Design review of the part shown in the three views and the two pictorial views. Dimensions are in mm from the part's minimum x, y and z. Coordinates: 2 decimals unless noted, no trailing zeros. Loops run counter-clockwise (first coordinate to the right, second up) from the corner with the lowest first, then second, coordinate; pieces in that order, holes last. Notation, with made-up numbers: (-6, 33) - (17, 33) arc R21 ccw to (17, 40) - close; hole circle Ø6 at (30.25, 76). An arc over 180 degrees is marked (long way). One line per question, with ' | ' between items.
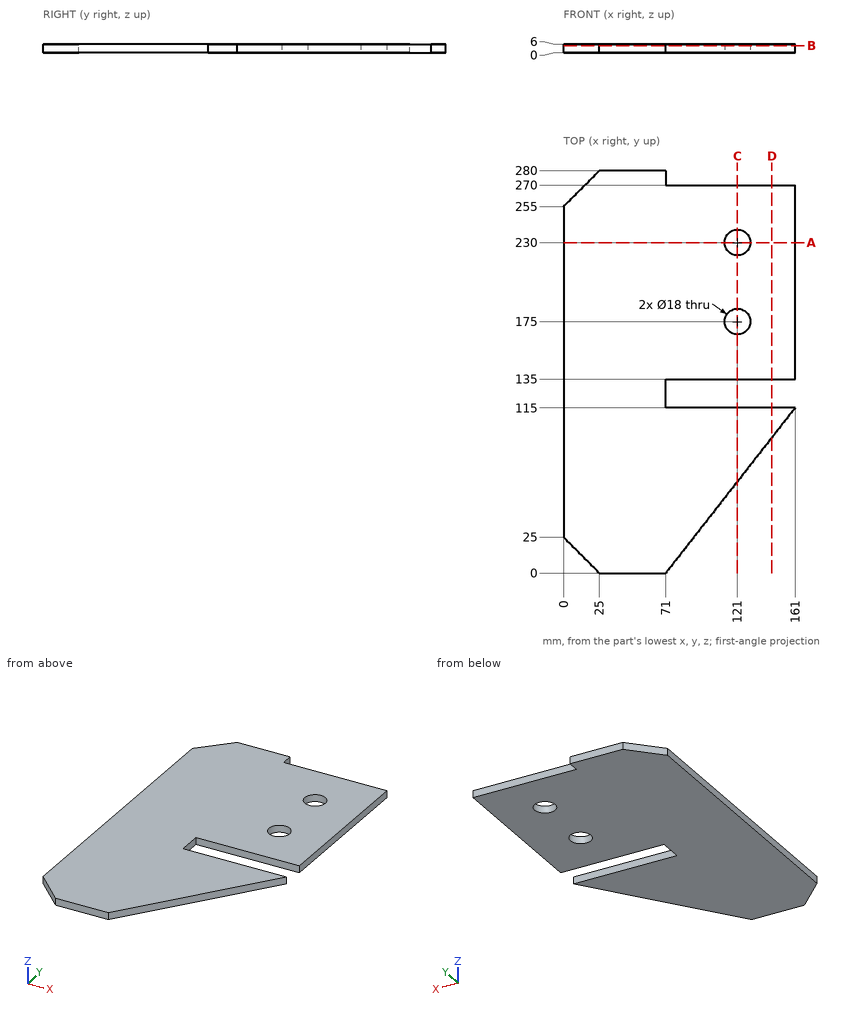
Q1. Take a section at B-B (z = 4.85). Give the boundary of the cut face in (x, y), plus the area to 3 significant figures.
Returned:
outline: (0, 25) - (25, 0) - (71, 0) - (161, 115) - (71, 115) - (71, 135) - (161, 135) - (161, 270) - (71, 270) - (71, 280) - (25, 280) - (0, 255) - close; hole circle Ø18 at (121, 175); hole circle Ø18 at (121, 230) | area: 36,100 mm²
Q2. For pin 1 (3 mm diameter, centred on x = 103, z = 4, fed in from +Y); pin 2 (2 mm diameter, centred on y = 57.5, z = 2.5, fed in from +X), all flat-tipped, find the tip position at first contact; note any pin that passes through.
Returned:
pin 1: stops at y = 270 | pin 2: stops at x = 116.78
Q3. To check wall thickness, follow line 1 along X through (y, z) = (175, 1.3); line 2 along Y through (x, z) = (121, 2.3); line 3 along X through (y, z) = (116, 0.95). State the ranges of each line that lie inside material, in increasing order.
Returned:
line 1: x = 0 to 112, 130 to 161 | line 2: y = 63.89 to 115, 135 to 166, 184 to 221, 239 to 270 | line 3: x = 0 to 71
Q4. Take a section at A-A (y = 230). Give the boundary of the cut face in (x, z), plus the area to 3 significant figures.
Returned:
outline: (0, 0) - (112, 0) - (112, 6) - (0, 6) - close; (130, 0) - (161, 0) - (161, 6) - (130, 6) - close | area: 858 mm²
Q5. Take a section at D-D (x = 145). Give the boundary of the cut face in (y, z), plus the area to 3 significant figures.
Returned:
outline: (94.56, 0) - (115, 0) - (115, 6) - (94.56, 6) - close; (135, 0) - (270, 0) - (270, 6) - (135, 6) - close | area: 933 mm²
Q6. Take a section at C-C (x = 121). Give the boundary of the cut face in (y, z), plus the area to 3 significant figures.
Returned:
outline: (63.89, 0) - (115, 0) - (115, 6) - (63.89, 6) - close; (135, 0) - (166, 0) - (166, 6) - (135, 6) - close; (184, 0) - (221, 0) - (221, 6) - (184, 6) - close; (239, 0) - (270, 0) - (270, 6) - (239, 6) - close | area: 901 mm²
